Model file for the job. Use its own axes, mm. A direction names the side the tool comes from. Round coordinates to 2 decimals unless told otherwise and drop trailing zeros. Loops run counter-clockwise (first coordinate to the right, second up) from the corner with the lowest first, then second, coordinate; pieces in that order, holes last. Notation, with made-up numbers: (51, 8) - (66, 8) arc R17 cw to (66, 14) - close; hole circle Ø2 at (40, -6). An arc over 180 degrees is marked (long way). Answer as a JSON object with one key per item and string values.
from build123d import *

# Parameters (mm, degrees)
SKETCH2_R           = 1
SKETCH2_R_2         = 5
BOSS_EXTRUDE1_DEPTH = 4


with BuildPart() as part:
    # Sketch2 → Boss-Extrude1 (new body)
    with BuildSketch(Plane.XY):
        with BuildLine():
            Line((10, -4.797958971), (10, -16.375449589))
            ThreePointArc((10, -16.375449589), (10.419623267, -19.898603621), (11.655015244, -23.224637999))
            Line((11.655015244, -23.224637999), (12.504814498, -24.880390098))
            ThreePointArc((12.504814498, -24.880390098), (12.432300446, -26.836100173), (10.725483197, -27.793615219))
            Line((10.725483197, -27.793615219), (-10.725483197, -27.793615219))
            ThreePointArc((-10.725483197, -27.793615219), (-12.432300446, -26.836100173), (-12.504814498, -24.880390098))
            Line((-12.504814498, -24.880390098), (-11.655015244, -23.224637999))
            ThreePointArc((-11.655015244, -23.224637999), (-10.419623267, -19.898603621), (-10, -16.375449589))
            Line((-10, -16.375449589), (-10, -4.797958971))
            ThreePointArc((-10, -4.797958971), (0, 11.091456635), (10, -4.797958971))
        make_face()
        with Locations((-8, -25.793615219)):
            Circle(SKETCH2_R, mode=Mode.SUBTRACT)
        with Locations((8, -25.793615219)):
            Circle(SKETCH2_R, mode=Mode.SUBTRACT)
        Circle(SKETCH2_R_2, mode=Mode.SUBTRACT)
        with Locations((0, -7.733897827)):
            Circle(SKETCH2_R, mode=Mode.SUBTRACT)
        with Locations((-6.697751988, 3.866948913)):
            Circle(SKETCH2_R, mode=Mode.SUBTRACT)
        with Locations((6.697751988, 3.866948913)):
            Circle(SKETCH2_R, mode=Mode.SUBTRACT)
        with BuildLine():
            Line((-2.92427416, -8.622098109), (-2.92427416, -24.622098109))
            ThreePointArc((-2.92427416, -24.622098109), (-4.92427416, -26.622098109), (-6.92427416, -24.622098109))
            Line((-6.92427416, -24.622098109), (-6.92427416, -8.622098109))
            ThreePointArc((-6.92427416, -8.622098109), (-4.92427416, -6.622098109), (-2.92427416, -8.622098109))
        make_face(mode=Mode.SUBTRACT)
        with BuildLine():
            Line((2.92427416, -8.622098109), (2.92427416, -24.622098109))
            ThreePointArc((2.92427416, -24.622098109), (4.92427416, -26.622098109), (6.92427416, -24.622098109))
            Line((6.92427416, -24.622098109), (6.92427416, -8.622098109))
            ThreePointArc((6.92427416, -8.622098109), (4.92427416, -6.622098109), (2.92427416, -8.622098109))
        make_face(mode=Mode.SUBTRACT)
    extrude(amount=BOSS_EXTRUDE1_DEPTH)


solid = part.part
1) Drop flat-ended pins along their axis: P1, Ø1.2, axis at y = -14, z = 2, coming from the +X side; P2, Ø1.2, axis at y = -13.5, z = 2.5, coming from the -X side; P3, Ø1.5, axis at x = 7, z = 2.5, coming from the +Y side. Give the stop position or say it passes through.
Values follow:
{"P1": "x = 10", "P2": "x = -10", "P3": "y = 9.16"}
2) Slice it at C-C on z = 3. Count the separate pieces of the cut face and the enclosed holes in it, then the cut area to 3 significant figures.
Values follow:
{"separate pieces": "1", "enclosed holes": "8", "area": "537 mm²"}
3) Slice it at A-A on x = 0. List the corners of the cut face in (y, z).
Values follow:
{"outline": "(-27.79, 0) - (-8.73, 0) - (-8.73, 4) - (-27.79, 4) - close; (-6.73, 0) - (-5, 0) - (-5, 4) - (-6.73, 4) - close; (5, 0) - (11.09, 0) - (11.09, 4) - (5, 4) - close"}
4) Tool access for faces 4 (the flat face through (10, -11, 2)), 5 (the flat face through (-10, -11, 2)), 6 (the cylindrical face through (-4.88, -26.62, 1.97)): list every direction of +Z, -Z, +X, -X, +Y, -Y with a clear straight run to the whole face (end or side of a thin tool).
Values follow:
{"face 4": "+Z, -Z, +X", "face 5": "+Z, -Z, -X", "face 6": "+Z, -Z"}
5) Two-plate mould, pull along X, no slides. Class faces 1 (the cylindrical face through (10.41, -19.85, 1.97)), 2 (the cylindrical face through (-10.431, -19.947, 1.972)), 3 (the cylindrical face through (7.2, 3, 2)): pulls with the +X half, pulls with the -X half, needs draft (parallel to the pull), parting line crosses it, or undercut.
Values follow:
{"face 1": "pulls with the +X half", "face 2": "pulls with the -X half", "face 3": "undercut"}
6) Probe probe 1 along Y at (x, z) = (0, 1.75); probe 2 along X at (y, z) = (-9.5, 2.9); probe 3 along X at (y, z) = (-21, 3.85). List the from-to ranges inside material, lowest first.
Values follow:
{"probe 1": "-27.79 to -8.73, -6.73 to -5, 5 to 11.09", "probe 2": "-10 to -6.92, -2.92 to 2.92, 6.92 to 10", "probe 3": "-10.73 to -6.92, -2.92 to 2.92, 6.92 to 10.73"}
7) Slice it at D-D on y = -22.5. List the corners of the cut face in (x, z).
Values follow:
{"outline": "(-11.31, 0) - (-6.92, 0) - (-6.92, 4) - (-11.31, 4) - close; (-2.92, 0) - (2.92, 0) - (2.92, 4) - (-2.92, 4) - close; (6.92, 0) - (11.31, 0) - (11.31, 4) - (6.92, 4) - close"}
8) Slice it at B-B on y = 0. List the corners of the cut face in (x, z), then the cut area to 3 significant figures.
Values follow:
{"outline": "(-11.09, 0) - (-5, 0) - (-5, 4) - (-11.09, 4) - close; (5, 0) - (11.09, 0) - (11.09, 4) - (5, 4) - close", "area": "48.7 mm²"}
